Autodesk Inventor part; units mm, degrees
ref_plane "YZ Plane" through (0, 0, 0) normal (1, 0, 0) x (0, 1, 0)
ref_plane "XZ Plane" through (0, 0, 0) normal (0, 1, 0) x (-1, 0, 0)
ref_plane "XY Plane" through (0, 0, 0) normal (0, 0, 1) x (1, 0, 0)
sketch "Sketch1" plane through (0, 0, 0) normal (0, 0, 1) x (1, 0, 0)
  line L0 (0, 0) -> (21.9725, 0)
  line L1 (40.4812, 0) -> (40.4812, 7.9375) construction
  line L2 (40.4812, 7.9375) -> (31.75, 7.9375)
  line L3 (0, 7.9375) -> (0, 6.35)
  line L4 (31.75, 0) -> (31.75, 7.9375) construction
  line L5 (31.75, 9.525) -> (22.225, 9.525)
  line L6 (22.225, 9.525) -> (22.225, 7.9375)
  line L7 (8.7312, 0) -> (8.7312, 17.4625) construction
  line L8 (8.7312, 17.4625) -> (0, 17.4625) construction
  line L9 (0, 17.4625) -> (0, 7.9375) construction
  line L10 (8.7312, 14.2875) -> (9.525, 14.2875) construction
  line L11 (9.525, 14.2875) -> (9.525, 7.9375) construction
  line L12 (9.525, 14.2875) -> (9.525, 27.94) construction
  line L13 (9.525, 27.94) -> (19.05, 27.94) construction
  line L14 (19.05, 27.94) -> (19.05, 7.9375) construction
  line L15 (22.225, 9.525) -> (22.225, 14.2875) construction
  line L16 (22.225, 14.2875) -> (21.4312, 14.2875) construction
  line L17 (21.4312, 14.2875) -> (21.4312, 7.9375) construction
  line L18 (21.4312, 14.2875) -> (21.4312, 17.4625) construction
  line L19 (21.4312, 17.4625) -> (14.2875, 17.4625) construction
  line L20 (14.2875, 17.4625) -> (14.2875, 0) construction
  line L21 (14.2875, 27.94) -> (14.2875, 17.4625) construction
  line L22 (14.1605, 27.94) -> (14.1605, 0) construction
  line L23 (11.9062, 27.94) -> (11.9062, 0) construction
  circle A0 centre (11.9062, 7.5565) radius 2.3813 construction
  line L24 (0, 5.5562) -> (6.2514, 5.5563) construction
  line L25 (0, 6.35) -> (6.2514, 6.35)
  line L26 (6.2514, 6.35) -> (6.2514, 5.5563)
  line L27 (6.2514, 5.5563) -> (6.2514, 0) construction
  line L28 (9.8391, 5.1753) -> (13.9734, 5.1753) construction
  line L29 (0, 3.175) -> (12.7284, 3.175)
  line L30 (6.2514, 5.5563) -> (19.0308, 5.5563)
  line L31 (0, 6.35) -> (0, 0) construction
  circle A1 centre (11.9062, 5.5562) radius 2.3813 construction
  circle A2 centre (11.9062, 5.8103) radius 2.3813 construction
  line L32 (14.2875, 8.1915) -> (9.525, 8.1915) construction
  line L33 (0, 3.175) -> (-5.4674, 3.175)
  line L34 (-5.4674, 3.175) -> (-5.4674, 2.3813)
  line L35 (-5.4674, 2.3813) -> (-10.4458, 2.3812)
  line L36 (-10.4458, 2.3812) -> (-10.4458, 0)
  line L37 (-10.4458, 0) -> (0, 0)
  line L38 (9.8391, 5.1753) -> (7.8389, 3.175) construction
  line L39 (12.7284, 3.175) -> (14.7286, 5.1753)
  line L40 (13.9734, 5.1753) -> (17.083, 0) construction
  line L41 (14.7286, 5.1753) -> (18.8629, 5.1753)
  line L42 (18.8629, 5.1753) -> (21.9725, 0)
  line L43 (19.0308, 5.5563) -> (22.3693, 0)
  line L44 (22.225, 5.5563) -> (31.75, 5.5563) construction
  line L45 (19.0308, 5.5563) -> (22.225, 5.5563) construction
  line L46 (22.225, 7.9375) -> (22.225, 0) construction
  line L47 (31.75, 7.9375) -> (31.75, 9.525)
  line L48 (31.75, 7.9375) -> (22.225, 7.9375) construction
  line L49 (22.225, 7.9375) -> (0, 7.9375)
  line L50 (31.75, 5.5563) -> (40.4812, 5.5563) construction
  line L51 (22.225, 0) -> (22.3693, 0) construction
  line L52 (22.3693, 0) -> (22.225, 0) construction
  line L53 (21.9725, 0) -> (22.3693, 0) construction
  line L54 (12.7284, 3.175) -> (40.4812, 3.175) construction
  line L55 (40.4812, 7.9375) -> (101.6, 7.9375)
  line L56 (101.6, 7.9375) -> (101.6, 0)
  line L57 (101.6, 0) -> (40.4812, 0)
  line L58 (22.3693, 0) -> (40.4812, 0)
  dimension "d0" = 7.9375
  dimension "d1" = 40.4813
  dimension "d2" = 9.525
  dimension "d3" = 8.7312
  dimension "d5" = 22.225
  dimension "d6" = 17.4625
  dimension "d7" = 8.7312
  dimension "d8" = 0.7937
  dimension "d9" = 14.2875
  dimension "d10" = 27.94
  dimension "d11" = 9.525
  dimension "d12" = 0.7937
  dimension "d14" = 7.1437
  dimension "d15" = 17.4625
  dimension "d16" = 0.127
  dimension "d17" = 4.7625
  dimension "d18" = 4.7625
  dimension "d19" = 5.5563
  dimension "d20" = 6.35
  dimension "d22" = 3.175
  dimension "d23" = 4.7625
  dimension "d24" = 4.7625
  dimension "d25" = 4.7625
  dimension "d26" = 0.254
  dimension "d27" = 2.0671
  dimension "d29" = 0.381
  dimension "d30" = 5.4673
  dimension "d31" = 4.9784
  dimension "d32" = 2.3813
  dimension "d33" = 45
  dimension "d34" = 45
  dimension "d35" = 0.0635
  dimension "d36" = 2.0671
  dimension "d37" = 59
  dimension "d38" = 4.1342
  dimension "d39" = 1.5875
  dimension "d40" = 0.3969
  dimension "d41" = 9.525
  dimension "d42" = 14.2875
  dimension "d43" = 61.1187
  dimension "d45" = 14.7287
  dimension "d46" = 9.8392
revolve "Revolution1" add sketch "Sketch1" angle 360 about axis through (101.6, 0, 0) along (-1, 0, 0) contours L55 L56 L57 L58 L43 L30 L26 L25 L3 L49 L6 L5 L47 L2
sketch "Sketch2" plane through (0, 0, 0) normal (0, 1, 0) x (-1, 0, 0)
  line L0 (-101.6, 7.9375) -> (-101.6, -7.9375)
  line L1 (-31.75, 7.9375) -> (-31.75, -7.9375)
  line L2 (-101.6, 0) -> (-53.975, 0) construction
  circle A0 centre (-79.375, 0) radius 3.175
  circle A1 centre (-53.975, 0) radius 3.175
  point P0 (0, 0)
  point P1 (-11.9062, 0)
  point P2 (-11.9062, 0)
  point P3 (-11.9062, 0)
  point P4 (-11.9062, 0)
  dimension "d59" = 25.4
  dimension "d60" = 22.225
  dimension "d61" = 6.35
  dimension "d62" = 6.35
hole "Hole1" at (11.9062, 0, 0) direction (0, 1, 0) diameter 4.8514 end through all
extrude "Extrusion1" cut sketch "Sketch2" along normal through all both and the other way through all
pattern_circular "Circular Pattern1" count 3 over 360 about axis through (-10, 0, 0) along (1, 0, 0) of "Hole1"
ref_plane "Work Plane1" through (14.7286, 0, 0) normal (-1, 0, 0) x (0, 0, 1)
ref_plane "Work Plane2" through (9.8391, 0, 0) normal (-1, 0, 0) x (0, 0, 1)
equation "\"d7\" = d3"
equation "\"d12\" = d8"
equation "\"d15\" = d6"
equation "\"d34\" = d33"
equation "\"d36\" = d27"
equation "\"d38\" = d27 + d36"
equation "\"d42\" = d9"
equation "\"d61\" = d62"
equation "\"d57\" = -d45"
equation "\"d58\" = -d46"
properties part number "Ball Shift"
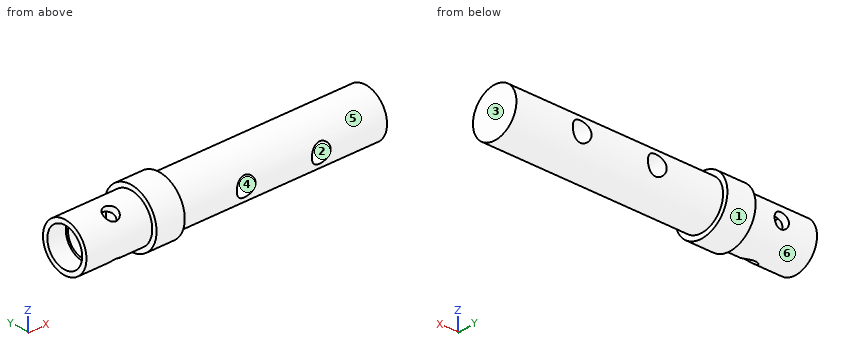
Read the model definition and answer for the solid it produces. Units are mm, in the model's axes. Face numbers are marked on the shaded views. A direction names the side the tool comes from. Coordinates: 2 decimals unless noted, no trailing zeros. Loops run counter-clockwise (first coordinate to the right, second up) from the corner with the lowest first, then second, coordinate; pieces in that order, holes last. Notation, with made-up numbers: (21.5, 34) -> (49.5, 34) arc R20 ccw to (49.5, 55) -> close; hole circle Ø2 at (-10.75, 61.5). An arc over 180 degrees is marked (long way). Return JSON: item names as keys, results as strings.
Item 1: Find the intervals of material crossed by probe 1 along X at (y, z) = (6.1, 0); probe 2 along X at (y, z) = (-7.75, 0); probe 3 along X at (y, z) = (7.15, 0), in increasing order.
Answers:
{"probe 1": "x = 6.25 to 9.48, 14.33 to 50.8, 57.15 to 76.2, 82.55 to 101.6", "probe 2": "x = 0 to 50.8, 57.15 to 76.2, 82.55 to 101.6", "probe 3": "x = 0 to 9.48, 14.33 to 50.8, 57.15 to 76.2, 82.55 to 101.6"}
Item 2: For a pull along X with two mould halves and no side action, classify the marked faces 1, 2 and 3 as +X half, -X half, draft (parallel to the pull), parting line (faces both ways), or undercut.
Answers:
{"face 1": "draft", "face 2": "undercut", "face 3": "+X half"}
Item 3: Find section B-B (x = 52.5). Determine the outline of the cut face in (y, z) (1 decimal), plus the area to 3 significant figures.
Answers:
{"outline": "(-7.4, -2.8) arc R7.9 ccw to (7.4, -2.8) -> close; (-7.4, 2.8) -> (7.4, 2.8) arc R7.9 ccw to start", "area": "111 mm2"}
Item 4: Flat-ended cylindrical pins translate along their axes: P1, Ø6, axis at x = 16, y = -5, coming from the +Z side; P2, Ø3, axis at x = 76, z = 6.5, coming from the +Y side; P3, Ø4, axis at y = 3, z = -1.5, coming from the -X side. Find the tip coordinate at first contact, or state that the pin passes through.
Answers:
{"P1": "stops at z = 7.68", "P2": "stops at y = 6.16", "P3": "stops at x = 19.15"}
Item 5: For the marked faces 4, 5 and 6, determine the directions among +Z, -Z, +X, -X, +Y, -Y from which every point of the face is accessible in a straight line to the end or side of a thin tool.
Answers:
{"face 4": "+Y, -Y", "face 5": "+X", "face 6": "-X"}
Item 6: Find section A-A (x = 36.5). Determine the outline of the cut face in (y, z) (1 decimal), plus the area to 3 significant figures.
Answers:
{"outline": "circle Ø15.9 at (0, 0)", "area": "198 mm2"}
